Geometry: final body of the model. Coordinates: model frame, mm. A direction names the side the tool comes from. Round coordinates to 2 decimals unless told otherwise and drop trailing zeros. Write each loop counter-clockwise with the first axis right and the second up, starting at its lowest first coordinate (ties: lowest second). Pieces come first, ordered by that corner, then holes.
from build123d import *

# Parameters (mm, degrees)
F0_R      = 19.05
F1_DEPTH  = 15.6718
F4_DEPTH  = 14.605
F5_R      = 17.4625
F6_DEPTH  = 19.05
F7_R      = 19.05
F7_R_2    = 15.5
F8_DEPTH  = 12.0396
F10_R     = 20.6375
F10_R_2   = 19.05
F11_DEPTH = 0.15875
F12_SIZE  = 1.58749
F13_R     = 15.24
F14_DEPTH = 19.05


# Not quite as in the source:
# - a fillet or chamfer is up to 0.001 mm smaller than in the source, because OpenCascade refuses the exact size


with BuildPart() as f1:
    # F0 (on Front) → F1 (new body, symmetric)
    with BuildSketch(Plane.XZ):
        Circle(F0_R)
    extrude(amount=F1_DEPTH, both=True)

    # F3 (on offset) → F4 (join)
    with BuildSketch(Plane.XZ.offset(10.9728)):
        with BuildLine():
            Line((-20.4035253035, 3.0988), (0, 0))
            Line((0, 0), (-16.6186535957, 12.2362886087))
            ThreePointArc((-16.6186535957, 12.2362886087), (-19.0665638522, 7.8976293354), (-20.4035253035, 3.0988))
        make_face()
        with BuildLine():
            Line((-12.2362886087, 16.6186535957), (0, 0))
            Line((0, 0), (-3.0988, 20.4035253035))
            ThreePointArc((-3.0988, 20.4035253035), (-7.8976293354, 19.0665638522), (-12.2362886087, 16.6186535957))
        make_face()
        with BuildLine():
            Line((3.0988, 20.4035253035), (0, 0))
            Line((0, 0), (12.2362886087, 16.6186535957))
            ThreePointArc((12.2362886087, 16.6186535957), (7.8976293354, 19.0665638522), (3.0988, 20.4035253035))
        make_face()
        with BuildLine():
            Line((0, 0), (20.4035253035, 3.0988))
            ThreePointArc((20.4035253035, 3.0988), (19.0665638522, 7.8976293354), (16.6186535957, 12.2362886087))
            Line((16.6186535957, 12.2362886087), (0, 0))
        make_face()
        with BuildLine():
            ThreePointArc((16.6186535957, -12.2362886087), (19.0665638522, -7.8976293354), (20.4035253035, -3.0988))
            Line((20.4035253035, -3.0988), (0, 0))
            Line((0, 0), (16.6186535957, -12.2362886087))
        make_face()
        with BuildLine():
            Line((12.2362886087, -16.6186535957), (0, 0))
            Line((0, 0), (3.0988, -20.4035253035))
            ThreePointArc((3.0988, -20.4035253035), (7.8976293354, -19.0665638522), (12.2362886087, -16.6186535957))
        make_face()
        with BuildLine():
            Line((-3.0988, -20.4035253035), (0, 0))
            Line((0, 0), (-12.2362886087, -16.6186535957))
            ThreePointArc((-12.2362886087, -16.6186535957), (-7.8976293354, -19.0665638522), (-3.0988, -20.4035253035))
        make_face()
        with BuildLine():
            Line((-16.6186535957, -12.2362886087), (0, 0))
            Line((0, 0), (-20.4035253035, -3.0988))
            ThreePointArc((-20.4035253035, -3.0988), (-19.0665638522, -7.8976293354), (-16.6186535957, -12.2362886087))
        make_face()
    extrude(amount=-F4_DEPTH)

    # F5 (on face) → F6 (cut)
    with BuildSketch(Plane.XZ.offset(15.6718)):
        Circle(F5_R)
    extrude(amount=-F6_DEPTH, mode=Mode.SUBTRACT)

    # F7 (on face) → F8 (cut)
    with BuildSketch(Plane(origin=(0, 15.6718, 0), x_dir=(-1, 0, 0), z_dir=(0, 1, 0))):
        Circle(F7_R)
        Circle(F7_R_2, mode=Mode.SUBTRACT)
    extrude(amount=-F8_DEPTH, mode=Mode.SUBTRACT)

    # F10 (on offset) → F11 (cut, symmetric)
    with BuildSketch(Plane.XZ.offset(3.6703)):
        Circle(F10_R)
        Circle(F10_R_2, mode=Mode.SUBTRACT)
    extrude(amount=F11_DEPTH, both=True, mode=Mode.SUBTRACT)

    # F12 (size 1.5875 in the source; OpenCascade refuses exactly that, so slightly less here)
    f12_edges = [f1.edges().sort_by_distance(p)[0] for p in [
        (-7.897629, -3.51155, 19.066564),
        (-7.897629, -3.82905, 19.066564),
        (-7.897629, -10.9728, 19.066564),
        (-7.897629, 3.6322, 19.066564),
        (-19.066564, 3.6322, 7.897629),
        (-19.066564, -3.51155, 7.897629),
        (-19.066564, -3.82905, 7.897629),
        (-19.066564, -10.9728, 7.897629),
        (-19.066564, -10.9728, -7.897629),
        (-19.066564, -3.82905, -7.897629),
        (-19.066564, -3.51155, -7.897629),
        (-19.066564, 3.6322, -7.897629),
        (-7.897629, -10.9728, -19.066564),
        (-7.897629, -3.82905, -19.066564),
        (-7.897629, -3.51155, -19.066564),
        (-7.897629, 3.6322, -19.066564),
        (7.897629, -3.82905, -19.066564),
        (7.897629, -10.9728, -19.066564),
        (7.897629, -3.51155, -19.066564),
        (7.897629, 3.6322, -19.066564),
        (19.066564, 3.6322, -7.897629),
        (19.066564, -3.51155, -7.897629),
        (19.066564, -3.82905, -7.897629),
        (19.066564, -10.9728, -7.897629),
        (19.066564, 3.6322, 7.897629),
        (19.066564, -3.51155, 7.897629),
        (19.066564, -3.82905, 7.897629),
        (19.066564, -10.9728, 7.897629),
        (7.897629, 3.6322, 19.066564),
        (7.897629, -3.51155, 19.066564),
        (7.897629, -3.82905, 19.066564),
        (7.897629, -10.9728, 19.066564),
    ]]
    chamfer(f12_edges, length=F12_SIZE)

    # F13 (on face) → F14 (join)
    with BuildSketch(Plane.XZ.offset(-3.3782)):
        with BuildLine():
            Line((1.5875, -15.7954255641), (-1.5875, -15.7954255641))
            ThreePointArc((-1.5875, -15.7954255641), (0, -15.875), (1.5875, -15.7954255641))
        make_face()
        with BuildLine():
            ThreePointArc((1.5875, -15.7954255641), (11.7732150983, -10.6492737428), (15.875, 0))
            ThreePointArc((15.875, 0), (-10.6492737428, 11.7732150983), (-1.5875, -15.7954255641))
            Line((-1.5875, -15.7954255641), (1.5875, -15.7954255641))
        make_face()
        Circle(F13_R, mode=Mode.SUBTRACT)
        with BuildLine():
            ThreePointArc((1.5875, -15.7954255641), (0, -15.875), (-1.5875, -15.7954255641))
            Line((-1.5875, -15.7954255641), (-1.5875, -17.0654255641))
            Line((-1.5875, -17.0654255641), (1.5875, -17.0654255641))
            Line((1.5875, -17.0654255641), (1.5875, -15.7954255641))
        make_face()
    extrude(amount=F14_DEPTH)


solid = f1.part
1) Reachability of faces 5 (the flat face through (-11.76, -7.45, -15.97)), 6 (the conical face through (-18.13, -2.91, 7.58)), 7 (the cylindrical face through (-13.858, -6.28, -10.626)) from +Z, -Z, +X, -X, +Y, -Y: full face, straight path, thin tool, end or side. Return the list, or none.
2) Section C-C on z = -14. Output: boundary loops of the cut face in (x, y), plus the area to 3 significant figures.
3) Section B-B on y = 1.5. State how many separate pieces and enclosed holes the cut face has, plus the area to 3 significant figures.
4) Draft query along X for faces 1 (the flat face through (-11.772, 0.01, 15.988)), 2 (the flat face through (-2.98, -7.45, 19.61)), 3 (the flat face through (11.772, 0.01, -15.988)), 4 (the cylindrical face through (-19.03, -8.3, 0.84)). Return one class per face: pulls with the +X half, pulls with the -X half, needs draft (parallel to the pull), parting line crosses it, or undercut.
5) First-contact query: P1, Ø3, axis at x = 10, y = 6.5, coming from the +Z side; P2, Ø3, axis at x = -2.5, y = 2, coming from the +Z side; P3, Ø1, axis at y = -6, z = -16.5, coming from the +X side; P4, Ø1, axis at x = 6.5, y = -2, coming from the -Z side. Flat tips, straight axial feed; report the tip coordinate or a pass-through.
6) Line query: probe 1 along X at (y, z) = (-13, -3); probe 2 along Z at (x, y) = (-14, 2). Output: solid intervals per line, ascending.
Filled in:
1. face 5: -X, +Y, -Y
1. face 6: +Z, -X
1. face 7: -Y
2. outline: (-12.92, -15.67) - (-10.44, -15.67) - (-10.44, 3.38) - (-7.48, 3.38) - (-7.48, -15.67) - (-6.02, -15.67) - (-6.02, 3.38) - (6.02, 3.38) - (6.02, -15.67) - (7.48, -15.67) - (7.48, 3.38) - (10.44, 3.38) - (10.44, -15.67) - (12.92, -15.67) - (12.92, 3.63) - (6.65, 3.63) - (6.65, 15.67) - (-6.65, 15.67) - (-6.65, 3.63) - (-12.92, 3.63) - close
2. area: 317 mm2
3. separate pieces: 2
3. enclosed holes: 2
3. area: 370 mm2
4. face 1: pulls with the -X half
4. face 2: undercut
4. face 3: pulls with the +X half
4. face 4: undercut
5. P1: stops at z = 12.96
5. P2: stops at z = 20.4
5. P3: stops at x = 12.24
5. P4: stops at z = -19.74
6. probe 1: x = -18.81 to -17.2, -15.59 to -14.94, 14.94 to 15.59, 17.2 to 18.81
6. probe 2: z = -12.92 to -10.44, -7.48 to -6.02, 6.02 to 7.48, 10.44 to 12.92
